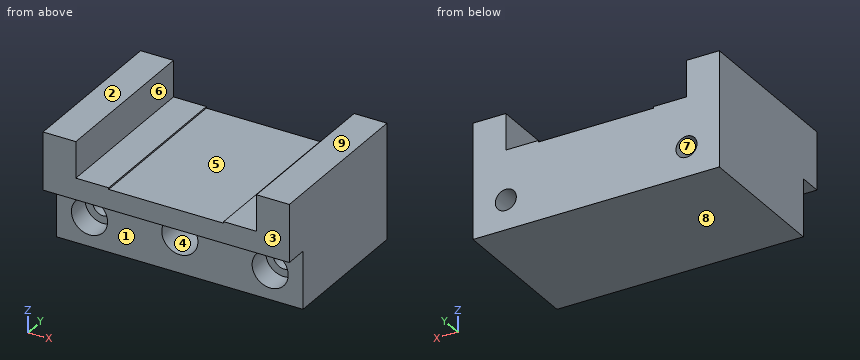
Autodesk Inventor part; units mm, degrees
ref_plane "YZ Plane" through (0, 0, 0) normal (1, 0, 0) x (0, 1, 0)
ref_plane "XZ Plane" through (0, 0, 0) normal (0, 1, 0) x (-1, 0, 0)
ref_plane "XY Plane" through (0, 0, 0) normal (0, 0, 1) x (1, 0, 0)
sketch "Sketch1" plane through (0, 0, 0) normal (0, 1, 0) x (-1, 0, 0)
  line L0 (-37.5, -17.5) -> (37.5, -17.5)
  line L1 (37.5, -17.5) -> (37.5, 17.5)
  line L2 (-37.5, 17.5) -> (-37.5, -17.5)
  line L3 (-37.5, -17.5) -> (37.5, 17.5) construction
  line L4 (37.5, -17.5) -> (-37.5, 17.5) construction
  line L5 (37.5, 17.5) -> (27.5, 17.5)
  line L6 (27.5, 17.5) -> (27.5, 6.5)
  line L7 (27.5, 6.5) -> (17.5, 6.5)
  line L8 (17.5, 6.5) -> (17.5, 6.0228)
  line L9 (17.5, 6.0228) -> (-17.5, 6.0228)
  line L10 (-17.5, 6.0228) -> (-17.5, 6.5)
  line L11 (-17.5, 6.5) -> (-27.5, 6.5)
  line L12 (-27.5, 6.5) -> (-27.5, 17.5)
  circle A0 centre (27.5, -8.5) radius 5.5
  circle A1 centre (-27.5, -8.5) radius 5.5
  circle A2 centre (0, -6.5) radius 5.5
  line L13 (37.5, 17.5) -> (27.5, 17.5)
  line L14 (-27.5, 17.5) -> (-37.5, 17.5)
  line L15 (-37.5, 1.5) -> (37.5, 1.5)
  line L16 (-37.5, 17.5) -> (-37.5, 1.5)
  line L17 (37.5, 1.5) -> (37.5, 17.5)
  line L18 (27.5, 17.5) -> (27.5, 6.5)
  line L19 (17.5, 6.5) -> (17.5, 6.0228)
  line L20 (-17.5, 6.0228) -> (-17.5, 6.5)
  line L21 (-27.5, 6.5) -> (-27.5, 17.5)
  line L22 (-37.5, 17.5) -> (-37.5, 1.5)
  point P0 (0, 0)
  point P1 (-32.5, 17.5)
  dimension "d0" = 75
  dimension "d1" = 35
  dimension "d2" = 10
  dimension "d3" = 11
  dimension "d4" = 10
  dimension "d5" = 35
  dimension "d6" = 10
  dimension "d7" = 11
  dimension "d8" = 11
  dimension "d10" = 11
  dimension "d12" = 27.5
  dimension "d13" = 27.5
  dimension "d41" = 16
extrude "Extrusion1" add sketch "Sketch1" along normal blind 7
sketch "Sketch2" plane through (0, 7, 0) normal (0, 1, 0) x (1, 0, 0)
  line L0 (-37.5, 17.5) -> (-37.5, -17.5)
  line L1 (-37.5, -17.5) -> (-37.5, 17.5)
  line L2 (37.5, 17.5) -> (-37.5, 17.5)
  line L3 (-37.5, 17.5) -> (37.5, 17.5)
  line L4 (37.5, -17.5) -> (37.5, 17.5)
  line L5 (37.5, 17.5) -> (37.5, -17.5)
  line L6 (27.5, -17.5) -> (37.5, -17.5)
  line L7 (37.5, -17.5) -> (27.5, -17.5)
  line L8 (27.5, -6.5) -> (27.5, -17.5)
  line L9 (27.5, -17.5) -> (27.5, -6.5)
  line L10 (17.5, -6.5) -> (27.5, -6.5)
  line L11 (27.5, -6.5) -> (17.5, -6.5)
  line L12 (17.5, -6.0228) -> (17.5, -6.5)
  line L13 (17.5, -6.5) -> (17.5, -6.0228)
  line L14 (-17.5, -6.0228) -> (17.5, -6.0228)
  line L15 (17.5, -6.0228) -> (-17.5, -6.0228)
  line L16 (-17.5, -6.0228) -> (-17.5, -6.5)
  line L17 (-27.5, -6.5) -> (-17.5, -6.5)
  line L18 (-17.5, -6.5) -> (-27.5, -6.5)
  line L19 (-27.5, -17.5) -> (-27.5, -6.5)
  line L20 (-27.5, -6.5) -> (-27.5, -17.5)
  line L21 (-37.5, -17.5) -> (-27.5, -17.5)
  line L22 (-27.5, -17.5) -> (-37.5, -17.5)
  circle A0 centre (27.5, 8.5) radius 3.2
  circle A1 centre (-27.5, 8.5) radius 3.2
  circle A2 centre (0, 6.5) radius 5.5
  point P0 (0, 0)
  point P1 (-32.5, -17.5)
  dimension "d17" = 6.4
  dimension "d24" = 6.4
  dimension "d25" = 27.5
  dimension "d26" = 27.5
  dimension "d27" = 26
  dimension "d28" = 26
  dimension "d29" = 11
  dimension "d30" = 24
extrude "Extrusion2" add sketch "Sketch2" along normal blind 13
sketch "Sketch3" plane through (0, 20, 0) normal (0, 1, 0) x (1, 0, 0)
  line L0 (-37.5, -17.5) -> (-27.5, -17.5)
  line L1 (-37.5, -17.5) -> (-27.5, -17.5)
  line L2 (-27.5, -17.5) -> (-27.5, -6.5)
  line L3 (-27.5, -17.5) -> (-27.5, -6.5)
  line L4 (-27.5, -6.5) -> (-17.5, -6.5)
  line L5 (-27.5, -6.5) -> (-17.5, -6.5)
  line L6 (-17.5, -6.5) -> (-17.5, -6.0228)
  line L7 (-17.5, -6.5) -> (-17.5, -6.0228)
  line L8 (-17.5, -6.0228) -> (17.5, -6.0228)
  line L9 (-17.5, -6.0228) -> (17.5, -6.0228)
  line L10 (17.5, -6.0228) -> (17.5, -6.5)
  line L11 (17.5, -6.0228) -> (17.5, -6.5)
  line L12 (17.5, -6.5) -> (27.5, -6.5)
  line L13 (17.5, -6.5) -> (27.5, -6.5)
  line L14 (27.5, -6.5) -> (27.5, -17.5)
  line L15 (27.5, -6.5) -> (27.5, -17.5)
  line L16 (27.5, -17.5) -> (37.5, -17.5)
  line L17 (27.5, -17.5) -> (37.5, -17.5)
  line L18 (37.5, 17.5) -> (-37.5, 17.5)
  line L19 (37.5, -17.5) -> (37.5, 17.5)
  line L20 (37.5, 17.5) -> (-37.5, 17.5)
  line L21 (-37.5, 17.5) -> (-37.5, -17.5)
  line L22 (-37.5, 17.5) -> (-37.5, -17.5)
  circle A0 centre (-27.5, 8.5) radius 3.2
  circle A1 centre (27.5, 8.5) radius 3.2
  point P0 (0, 0)
  point P1 (0, -6.0228)
  point P2 (0, -6.0228)
  dimension "d33" = 6.4
  dimension "d34" = 6.4
  dimension "d35" = 26
  dimension "d36" = 27.5
  dimension "d37" = 27.5
extrude "Extrusion3" add sketch "Sketch3" along normal blind 23
sketch "Sketch5" plane through (0, 0, 0) normal (0, -1, 0) x (1, 0, 0)
  line L0 (37.5, 17.5) -> (37.5, -17.5)
  line L1 (37.5, 0) -> (-37.5, 0)
  line L2 (-37.5, -17.5) -> (-37.5, 17.5)
  line L3 (-37.5, 17.5) -> (-27.5, 17.5)
  line L4 (-37.5, 17.5) -> (-27.5, 17.5)
  line L5 (-27.5, 17.5) -> (-27.5, 6.5)
  line L6 (-27.5, 17.5) -> (-27.5, 6.5)
  line L7 (-27.5, 6.5) -> (-17.5, 6.5)
  line L8 (-27.5, 6.5) -> (-17.5, 6.5)
  line L9 (-17.5, 6.0228) -> (17.5, 6.0228)
  line L10 (-17.5, 6.5) -> (-17.5, 6.0228)
  line L11 (-17.5, 6.0228) -> (17.5, 6.0228)
  line L12 (17.5, 6.0228) -> (17.5, 6.5)
  line L13 (17.5, 6.5) -> (27.5, 6.5)
  line L14 (17.5, 6.5) -> (27.5, 6.5)
  line L15 (27.5, 6.5) -> (27.5, 17.5)
  line L16 (27.5, 6.5) -> (27.5, 17.5)
  line L17 (27.5, 17.5) -> (37.5, 17.5)
  line L18 (27.5, 17.5) -> (37.5, 17.5)
  line L19 (37.5, 17.5) -> (37.5, 0)
  point P0 (0, 0)
extrude "Extrusion4" add sketch "Sketch5" along normal blind 7
properties part number "Lose backe" material "Steel"
The listing builds one solid part. Answer for the finished solid, in the listing's coordinates (mm). Face numbers are marked on the shaded views. A direction names the side the tool comes from. Round coordinates to 2 decimals unless told otherwise and drop trailing zeros. Write each loop counter-clockwise with the first axis right and the second up, starting at its lowest first coordinate (ties: lowest second). Pieces come first, ordered by that corner, then holes. Notation, with made-up numbers: (64, 42) -> (115, 42) arc R21 cw to (115, 46) -> close; hole circle Ø7 at (17, 21). An arc over 180 degrees is marked (long way). Answer as a JSON object with one key per item and string values. Group by question number.
Q1. Section C-C (z = -8.5) is taken. Write down the section's boundary in (x, y), plus the area to 3 significant figures.
Q2. Each of these flat-tipped pins is pushed along its axis until it touches: pin 1 Ø8 at (x, y) = (24, 21) entering from +Z; pin 2 Ø14 at (x, z) = (17, -10.5) entering from -Y; pin 3 Ø9 at (x, z) = (27.5, -8.5) entering from -Y; pin 4 Ø8 at (x, y) = (-2, 31) entering from +Z. Where does it stop, or does it pass through?
Q3. Straight lines are drawn through the part: line 1 along X through (y, z) = (39, -8); line 2 along X through (y, z) = (-1, 10.5); line 3 along Z through (x, y) = (0, 11). For each, find the intervals that lie inside material, in ascending order.
Q4. Section B-B (y = 14.5) is taken. Write down the section's boundary in (x, z), plus the area to 3 significant figures.
Q5. Section A-A (y = 30.5) is taken. Write down the section's boundary in (x, z), plus the area to 3 significant figures.
Q6. Section D-D (x = 19.5) is taken. Write down the section's boundary in (y, z).
Q7. Determine the mould class of the marked faces 6, 7, 8 and 9 for opening direction Z: pulls with the +Z half, pulls with the -Z half, needs draft (parallel to the pull), parting line crosses it, or undercut.
Q8. Which of the six approach directions +Z, -Z, +X, -X, +Y, -Y give full straight-line access (tool end or side, diameter ignored) to the marked faces 1, 2, 3, 4 and 5?
Check values:
{
 "1": {"outline": "(-37.5, 0) -> (-33, 0) -> (-33, 7) -> (-30.7, 7) -> (-30.7, 43) -> (-37.5, 43) -> close; (-24.3, 7) -> (-22, 7) -> (-22, 0) -> (-5.12, 0) -> (-5.12, 20) -> (5.12, 20) -> (5.12, 0) -> (22, 0) -> (22, 7) -> (24.3, 7) -> (24.3, 43) -> (-24.3, 43) -> close; (30.7, 7) -> (33, 7) -> (33, 0) -> (37.5, 0) -> (37.5, 43) -> (30.7, 43) -> close", "area": "2,410 mm^2"},
 "2": {"pin 1": "z = 17.5", "pin 2": "y = 0", "pin 3": "y = 7", "pin 4": "z = 6.02"},
 "3": {"line 1": "-37.5 to -30.66, -24.34 to 24.34, 30.66 to 37.5", "line 2": "-37.5 to -27.5, 27.5 to 37.5", "line 3": "-17.5 to -12, -1 to 6.02"},
 "4": {"outline": "(-37.5, -17.5) -> (37.5, -17.5) -> (37.5, 17.5) -> (27.5, 17.5) -> (27.5, 6.5) -> (17.5, 6.5) -> (17.5, 6.02) -> (-17.5, 6.02) -> (-17.5, 6.5) -> (-27.5, 6.5) -> (-27.5, 17.5) -> (-37.5, 17.5) -> close; hole circle Ø6.4 at (-27.5, -8.5); hole circle Ø11 at (0, -6.5); hole circle Ø6.4 at (27.5, -8.5)", "area": "1,840 mm^2"},
 "5": {"outline": "(-37.5, -17.5) -> (37.5, -17.5) -> (37.5, 17.5) -> (27.5, 17.5) -> (27.5, 6.5) -> (17.5, 6.5) -> (17.5, 6.02) -> (-17.5, 6.02) -> (-17.5, 6.5) -> (-27.5, 6.5) -> (-27.5, 17.5) -> (-37.5, 17.5) -> close; hole circle Ø6.4 at (-27.5, -8.5); hole circle Ø6.4 at (27.5, -8.5)", "area": "1,940 mm^2"},
 "6": {"outline": "(-7, 0) -> (0, 0) -> (0, -17.5) -> (43, -17.5) -> (43, 6.5) -> (-7, 6.5) -> close"},
 "7": {"face 6": "needs draft", "face 7": "undercut", "face 8": "pulls with the -Z half", "face 9": "pulls with the +Z half"},
 "8": {"face 1": "-Z, +X, -X, -Y", "face 2": "+Z, +X, -X, +Y, -Y", "face 3": "+Z, -Z, +X, -X, -Y", "face 4": "-Y", "face 5": "+Z, +Y, -Y"}
}
